For this review, use the dimensioned drawing (mm, ordinates from the lowest corner) and the shaded views. A direction names the side the tool comes from. Give positions to 0.01 mm unless a question says otherwise; leave off trailing zeros. Order: outer loops, then holes, each group sorted by start corner. A loop starts at its lowest first (then second) coordinate and runs counter-clockwise, first axis right, second up. Notation, with made-up numbers: M -4.5,-7 L 15.5,-7 A22 ccw 15.5,10 Z; hole C -12,-7.75 d2. An arc over 180 degrees is marked long. Answer as CSV lines item,"result". Start each with the question number.
1. Mouldability with a two-part tool opening along X and no side actions: class the marked faces 1, 2, 3 and 4 as pulls with the +X half, pulls with the -X half, needs draft (parallel to the pull), parting line crosses it, or undercut.
2. We need section D-D, the plane z = 15.5. Give the boundary of the cut face in (x, y), and give its area (3 significant figures).
3. We need section A-A, the plane y = 11. Give the boundary of the cut face in (x, z).
4. We need section C-C, the plane z = 2.5. Give the boundary of the cut face in (x, y), and give its area (3 significant figures).
5. We need section B-B, the plane x = 25.5. Give the boundary of the cut face in (y, z).
6. Clearance check with flat-ended pins moving along their axes: P1, Ø0.8, axis at y = 3, z = 4.5, coming from the +X side; P2, Ø3.5, axis at x = 43.5, y = 18.5, coming from the -Z side; P3, Ø1.5, axis at y = 15.5, z = 21.5, coming from the +X side. State where each tip first meets the part, or that it passes through.
7. For line 1 along Y through (x, z) = (3.5, 11.9); line 2 along Z through (x, y) = (42, 7.25); line 3 along Z through (x, y) = (35, 15), list the stretches that pass through material, from the lowest coordinate up.
8. Machinability: for the marked faces 5, 6, 7 and 8, which of the approach directions +Z, -Z, +X, -X, +Y, -Y give a long, thin tool a straight path to every point of the face, cutting with its end or side? Answer none if there is none.
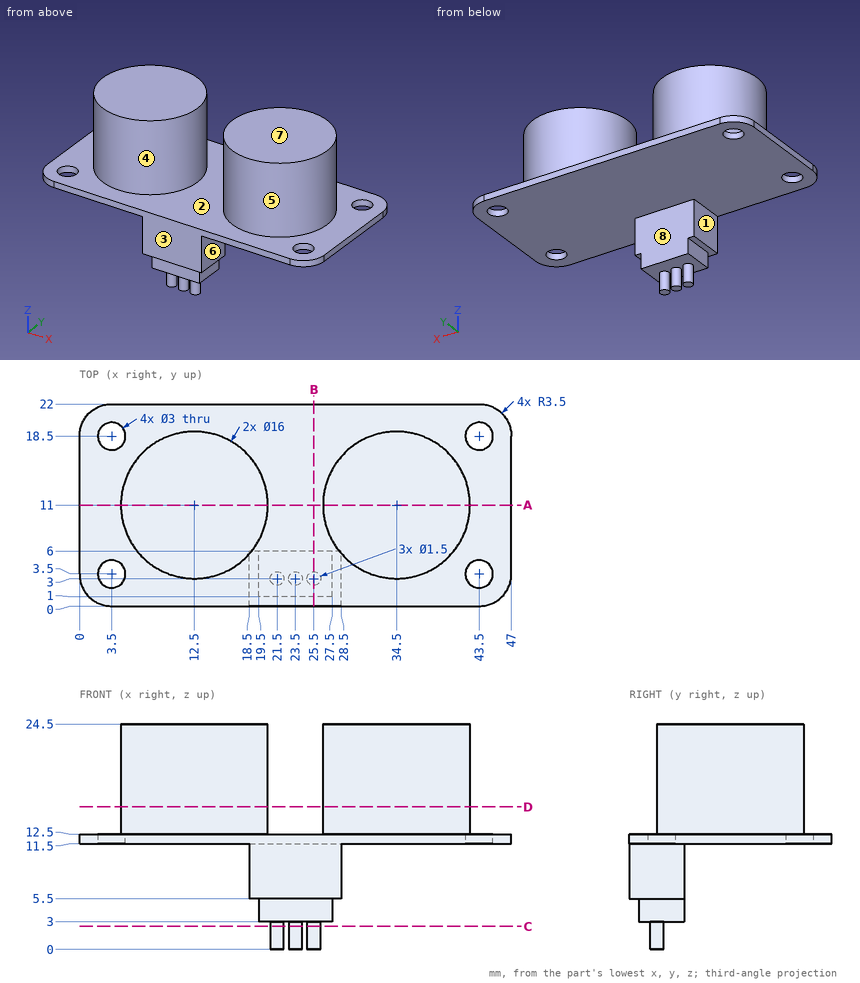
Result set:
1,face 1,"pulls with the -X half"
1,face 2,"undercut"
1,face 3,"needs draft"
1,face 4,"undercut"
2,outline,"C 12.5,11 d16; C 34.5,11 d16"
2,area,"402 mm2"
3,outline,"M 0,11.5 L 47,11.5 L 47,12.5 L 42.5,12.5 L 42.5,24.5 L 26.5,24.5 L 26.5,12.5 L 20.5,12.5 L 20.5,24.5 L 4.5,24.5 L 4.5,12.5 L 0,12.5 Z"
4,outline,"C 21.5,3 d1.5; C 23.5,3 d1.5; C 25.5,3 d1.5"
4,area,"5.30 mm2"
5,outline,"M 0,5.5 L 1,5.5 L 1,3 L 2.25,3 L 2.25,0 L 3.75,0 L 3.75,3 L 6,3 L 6,11.5 L 22,11.5 L 22,12.5 L 0,12.5 Z"
6,P1,"x = 27.5"
6,P2,"z = 11.5"
6,P3,"x = 41.57"
7,line 1,"0 to 2, 5 to 17, 20 to 22"
7,line 2,"11.5 to 12.5"
7,line 3,"11.5 to 24.5"
8,face 5,"+Z"
8,face 6,"-Z, +X, +Y, -Y"
8,face 7,"+Z, +X, -X, +Y, -Y"
8,face 8,"-Z, +X, -X, +Y"
